Source: three-view drawing plus pictorial views. Frame: mm from the lowest corner of the part. A direction names the side the tool comes from. Give positions to 0.01 mm unless a question says otherwise; leave off trailing zeros. Loops run counter-clockwise (first coordinate to the right, second up) from the corner with the lowest first, then second, coordinate; pieces in that order, holes last. Notation, with made-up numbers: (-16, 85) - (19, 85) arc R9 ccw to (19, 92) - close; hole circle Ø1 at (4, 71.25). An arc over 180 degrees is marked (long way). Answer as a JSON object with one key per item and string values.
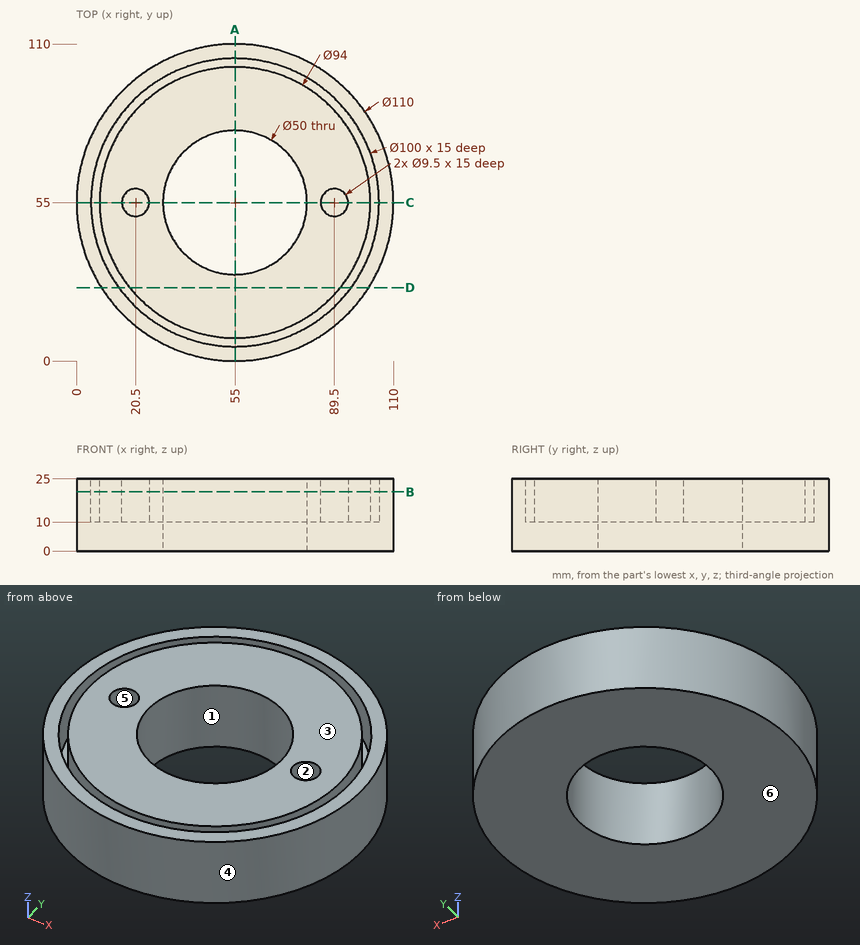
Item 1: Material intervals for line 1 (X direction, y = 75.5, z = 13); line 2 (X direction, y = 85, z = 24); line 3 (X direction, y = 65, z = 17.5), sorted ascending. Write a range as [from, to].
Geometry check:
{"line 1": "x = [3.96, 9.4], [12.71, 40.69], [69.31, 97.29], [100.6, 106.04]", "line 2": "x = [8.9, 15], [18.82, 91.18], [95, 101.1]", "line 3": "x = [0.92, 6.01], [9.08, 32.09], [77.91, 100.92], [103.99, 109.08]"}
Item 2: Cut plane D-D (y = 25.5). Return loops of the section in (x, z).
Geometry check:
{"outline": "(8.58, 0) - (101.42, 0) - (101.42, 25) - (95.37, 25) - (95.37, 10) - (91.59, 10) - (91.59, 25) - (18.41, 25) - (18.41, 10) - (14.63, 10) - (14.63, 25) - (8.58, 25) - close"}
Item 3: Cut plane A-A (x = 55). Return loops of the section in (y, z).
Geometry check:
{"outline": "(0, 0) - (30, 0) - (30, 25) - (8, 25) - (8, 10) - (5, 10) - (5, 25) - (0, 25) - close; (80, 0) - (110, 0) - (110, 25) - (105, 25) - (105, 10) - (102, 10) - (102, 25) - (80, 25) - close"}
Item 4: Mould query, pull axis Y, two halves, no side actions, for the marked faces 1, 2, 3 and 4. Classes: released by +Y, released by -Y, zero draft, split by the parting line, or undercut.
Geometry check:
{"face 1": "undercut", "face 2": "undercut", "face 3": "zero draft", "face 4": "split by the parting line"}
Item 5: Contact query for flat-ended pins moving along their axis: P1, Ø5.5, axis at x = 89.5, y = 55, coming from the +Z side; P2, Ø7.5, axis at x = 89.5, y = 53.5, coming from the +Z side; P3, Ø2, axis at x = 49.5, z = 4.5, coming from the +Y side; P4, Ø8, axis at x = 66.5, z = 18, coming from the -Y side. Output: stop coordinate, or through.
Geometry check:
{"P1": "stops at z = 10", "P2": "stops at z = 25", "P3": "stops at y = 109.82", "P4": "stops at y = 0.51"}
Item 6: Cut plane B-B (z = 20.5). Return loops of the section in (x, y), then the cut area to 3 significant figures.
Geometry check:
{"outline": "circle Ø110 at (55, 55); circle Ø94 at (55, 55); hole circle Ø100 at (55, 55); hole circle Ø9.5 at (20.5, 55); hole circle Ø50 at (55, 55); hole circle Ø9.5 at (89.5, 55)", "area": "6,480 mm2"}
Item 7: Access query for the marked faces 5 and 6. Directions: +Z, -Z, +X, -X, +Y, -Y. A direction counts if a zero-diameter tool reaches every point of the face in a straight line with its end or side. Return the directions, or none.
Geometry check:
{"face 5": "+Z", "face 6": "-Z, +X, -X, +Y, -Y"}
Item 8: Cut plane C-C (y = 55). Return loops of the section in (x, z), then the cut area to 4 significant figures.
Geometry check:
{"outline": "(0, 0) - (30, 0) - (30, 25) - (25.25, 25) - (25.25, 10) - (15.75, 10) - (15.75, 25) - (8, 25) - (8, 10) - (5, 10) - (5, 25) - (0, 25) - close; (80, 0) - (110, 0) - (110, 25) - (105, 25) - (105, 10) - (102, 10) - (102, 25) - (94.25, 25) - (94.25, 10) - (84.75, 10) - (84.75, 25) - (80, 25) - close", "area": "1,125 mm2"}
